Geometry: final body of the model. Coordinates: model frame, mm. Round coordinates to 2 decimals unless told otherwise and drop trailing zeros. Loops run counter-clockwise (first coordinate to the right, second up) from the corner with the lowest first, then second, coordinate; pieces in that order, holes last. Notation, with made-up numbers: (59.5, 2) - (75.5, 2) arc R25 cw to (75.5, 31) - close; hole circle Ø7 at (26.5, 39.25). An arc over 180 degrees is marked (long way). Use CSV: the item, a comma, the result in double quotes.
from build123d import *

# Parameters (mm, degrees)
SKETCH1_R           = 2.25
BOSS_EXTRUDE1_DEPTH = 2.15
SKETCH2_W           = 1.55
SKETCH2_H           = 4.8
CUT_EXTRUDE1_DEPTH  = 53


with BuildPart() as part:
    # Sketch1 → Boss-Extrude1 (new body)
    with BuildSketch(Plane.XY):
        with BuildLine():
            Line((2.398752887, -11.327345722), (26.384379929, -11.327345722))
            Line((26.384379929, -11.327345722), (26.384379929, 8.672654278))
            Line((26.384379929, 8.672654278), (26.024379959, 8.672654278))
            Line((26.024379959, 8.672654278), (24.744379959, 8.672654278))
            Line((24.744379959, 8.672654278), (24.744379959, 6.172654278))
            ThreePointArc((24.744379959, 6.172654278), (24.384379958, 5.812654278), (24.024379958, 6.172654278))
            Line((24.024379958, 6.172654278), (24.024379958, 8.672654278))
            Line((24.024379958, 8.672654278), (22.744379958, 8.672654278))
            Line((22.744379958, 8.672654278), (22.744379958, 6.172654278))
            ThreePointArc((22.744379958, 6.172654278), (22.384379957, 5.812654278), (22.024379957, 6.172654278))
            Line((22.024379957, 6.172654278), (22.024379957, 8.672654278))
            Line((22.024379957, 8.672654278), (20.744379957, 8.672654278))
            Line((20.744379957, 8.672654278), (20.744379957, 6.172654278))
            ThreePointArc((20.744379957, 6.172654278), (20.384379956, 5.812654278), (20.024379956, 6.172654278))
            Line((20.024379956, 6.172654278), (20.024379956, 8.672654278))
            Line((20.024379956, 8.672654278), (18.744379956, 8.672654278))
            Line((18.744379956, 8.672654278), (18.744379956, 6.172654278))
            ThreePointArc((18.744379956, 6.172654278), (18.384379955, 5.812654278), (18.024379955, 6.172654278))
            Line((18.024379955, 6.172654278), (18.024379955, 8.672654278))
            Line((18.024379955, 8.672654278), (16.744379955, 8.672654278))
            Line((16.744379955, 8.672654278), (16.744379955, 6.172654278))
            ThreePointArc((16.744379955, 6.172654278), (16.384379953, 5.812654278), (16.024379953, 6.172654278))
            Line((16.024379953, 6.172654278), (16.024379953, 8.672654278))
            Line((16.024379953, 8.672654278), (14.744379953, 8.672654278))
            Line((14.744379953, 8.672654278), (14.744379953, 6.172654278))
            ThreePointArc((14.744379953, 6.172654278), (14.384379952, 5.812654278), (14.024379952, 6.172654278))
            Line((14.024379952, 6.172654278), (14.024379952, 8.672654278))
            Line((14.024379952, 8.672654278), (12.744379952, 8.672654278))
            Line((12.744379952, 8.672654278), (12.744379952, 6.172654278))
            ThreePointArc((12.744379952, 6.172654278), (12.384379951, 5.812654278), (12.024379951, 6.172654278))
            Line((12.024379951, 6.172654278), (12.024379951, 8.672654278))
            Line((12.024379951, 8.672654278), (10.744379951, 8.672654278))
            Line((10.744379951, 8.672654278), (10.744379951, 6.172654278))
            ThreePointArc((10.744379951, 6.172654278), (10.38437995, 5.812654278), (10.02437995, 6.172654278))
            Line((10.02437995, 6.172654278), (10.02437995, 8.672654278))
            Line((10.02437995, 8.672654278), (8.74437995, 8.672654278))
            Line((8.74437995, 8.672654278), (8.74437995, 6.172654278))
            ThreePointArc((8.74437995, 6.172654278), (8.384379949, 5.812654278), (8.024379949, 6.172654278))
            Line((8.024379949, 6.172654278), (8.024379949, 8.672654278))
            Line((8.024379949, 8.672654278), (6.744379949, 8.672654278))
            Line((6.744379949, 8.672654278), (6.744379949, 6.172654278))
            ThreePointArc((6.744379949, 6.172654278), (6.384379947, 5.812654278), (6.024379947, 6.172654278))
            Line((6.024379947, 6.172654278), (6.024379947, 8.672654278))
            Line((6.024379947, 8.672654278), (4.744379947, 8.672654278))
            Line((4.744379947, 8.672654278), (4.744379947, 6.172654278))
            ThreePointArc((4.744379947, 6.172654278), (4.384379946, 5.812654278), (4.024379946, 6.172654278))
            Line((4.024379946, 6.172654278), (4.024379946, 8.672654278))
            Line((4.024379946, 8.672654278), (2.744379946, 8.672654278))
            Line((2.744379946, 8.672654278), (2.744379946, 6.172654278))
            ThreePointArc((2.744379946, 6.172654278), (2.384379945, 5.812654278), (2.024379945, 6.172654278))
            Line((2.024379945, 6.172654278), (2.024379945, 8.672654278))
            Line((2.024379945, 8.672654278), (0.744379945, 8.672654278))
            Line((0.744379945, 8.672654278), (0.744379945, 6.172654278))
            ThreePointArc((0.744379945, 6.172654278), (0.384379944, 5.812654278), (0.024379944, 6.172654278))
            Line((0.024379944, 6.172654278), (0.024379944, 8.672654278))
            Line((0.024379944, 8.672654278), (-1.255620056, 8.672654278))
            Line((-1.255620056, 8.672654278), (-1.255620056, 6.172654278))
            ThreePointArc((-1.255620056, 6.172654278), (-1.615620057, 5.812654278), (-1.975620057, 6.172654278))
            Line((-1.975620057, 6.172654278), (-1.975620057, 8.672654278))
            Line((-1.975620057, 8.672654278), (-3.255620057, 8.672654278))
            Line((-3.255620057, 8.672654278), (-3.255620057, 6.172654278))
            ThreePointArc((-3.255620057, 6.172654278), (-3.615620059, 5.812654278), (-3.975620059, 6.172654278))
            Line((-3.975620059, 6.172654278), (-3.975620059, 8.672654278))
            Line((-3.975620059, 8.672654278), (-5.255620059, 8.672654278))
            Line((-5.255620059, 8.672654278), (-5.255620059, 6.172654278))
            ThreePointArc((-5.255620059, 6.172654278), (-5.61562006, 5.812654278), (-5.97562006, 6.172654278))
            Line((-5.97562006, 6.172654278), (-5.97562006, 8.672654278))
            Line((-5.97562006, 8.672654278), (-7.25562006, 8.672654278))
            Line((-7.25562006, 8.672654278), (-7.25562006, 6.172654278))
            ThreePointArc((-7.25562006, 6.172654278), (-7.615620061, 5.812654278), (-7.975620061, 6.172654278))
            Line((-7.975620061, 6.172654278), (-7.975620061, 8.672654278))
            Line((-7.975620061, 8.672654278), (-9.255620061, 8.672654278))
            Line((-9.255620061, 8.672654278), (-9.255620061, 6.172654278))
            ThreePointArc((-9.255620061, 6.172654278), (-9.615620062, 5.812654278), (-9.975620062, 6.172654278))
            Line((-9.975620062, 6.172654278), (-9.975620062, 8.672654278))
            Line((-9.975620062, 8.672654278), (-11.255620062, 8.672654278))
            Line((-11.255620062, 8.672654278), (-11.255620062, 6.172654278))
            ThreePointArc((-11.255620062, 6.172654278), (-11.615620063, 5.812654278), (-11.975620063, 6.172654278))
            Line((-11.975620063, 6.172654278), (-11.975620063, 8.672654278))
            Line((-11.975620063, 8.672654278), (-13.255620063, 8.672654278))
            Line((-13.255620063, 8.672654278), (-13.255620063, 6.172654278))
            ThreePointArc((-13.255620063, 6.172654278), (-13.615620065, 5.812654278), (-13.975620065, 6.172654278))
            Line((-13.975620065, 6.172654278), (-13.975620065, 8.672654278))
            Line((-13.975620065, 8.672654278), (-15.255620065, 8.672654278))
            Line((-15.255620065, 8.672654278), (-15.255620065, 6.172654278))
            ThreePointArc((-15.255620065, 6.172654278), (-15.615620066, 5.812654278), (-15.975620066, 6.172654278))
            Line((-15.975620066, 6.172654278), (-15.975620066, 8.672654278))
            Line((-15.975620066, 8.672654278), (-17.255620066, 8.672654278))
            Line((-17.255620066, 8.672654278), (-17.255620066, 6.172654278))
            ThreePointArc((-17.255620066, 6.172654278), (-17.615620067, 5.812654278), (-17.975620067, 6.172654278))
            Line((-17.975620067, 6.172654278), (-17.975620067, 8.672654278))
            Line((-17.975620067, 8.672654278), (-19.255620067, 8.672654278))
            Line((-19.255620067, 8.672654278), (-19.255620067, 6.172654278))
            ThreePointArc((-19.255620067, 6.172654278), (-19.615620068, 5.812654278), (-19.975620068, 6.172654278))
            Line((-19.975620068, 6.172654278), (-19.975620068, 8.672654278))
            Line((-19.975620068, 8.672654278), (-21.255620068, 8.672654278))
            Line((-21.255620068, 8.672654278), (-21.255620068, 6.172654278))
            ThreePointArc((-21.255620068, 6.172654278), (-21.615620069, 5.812654278), (-21.975620069, 6.172654278))
            Line((-21.975620069, 6.172654278), (-21.975620069, 8.672654278))
            Line((-21.975620069, 8.672654278), (-23.255620069, 8.672654278))
            Line((-23.255620069, 8.672654278), (-23.255620069, 6.172654278))
            ThreePointArc((-23.255620069, 6.172654278), (-23.615620071, 5.812654278), (-23.975620071, 6.172654278))
            Line((-23.975620071, 6.172654278), (-23.975620071, 8.672654278))
            Line((-23.975620071, 8.672654278), (-25.615620071, 8.672654278))
            Line((-25.615620071, 8.672654278), (-25.615620071, -11.327345722))
            Line((-25.615620071, -11.327345722), (-1.621247113, -11.327345722))
            Line((-1.621247113, -11.327345722), (-1.621247113, -7.327345722))
            ThreePointArc((-1.621247113, -7.327345722), (0.373417474, -5.293808364), (2.398752887, -7.296800492))
            Line((2.398752887, -7.296800492), (2.398752887, -11.327345722))
        make_face()
        with Locations((-19.615620071, -5.327345722)):
            Circle(SKETCH1_R, mode=Mode.SUBTRACT)
        with Locations((-9.615620071, -5.327345722)):
            Circle(SKETCH1_R, mode=Mode.SUBTRACT)
        with Locations((10.384379929, -5.327345722)):
            Circle(SKETCH1_R, mode=Mode.SUBTRACT)
        with Locations((20.384379929, -5.327345722)):
            Circle(SKETCH1_R, mode=Mode.SUBTRACT)
    extrude(amount=BOSS_EXTRUDE1_DEPTH)

    # Sketch2 → Cut-Extrude1 (cut, through all)
    with BuildSketch(Plane.ZY.offset(25.615620071)):
        with Locations((1.375, 6.272654278)):
            Rectangle(SKETCH2_W, SKETCH2_H)
    extrude(amount=-CUT_EXTRUDE1_DEPTH, mode=Mode.SUBTRACT)


solid = part.part
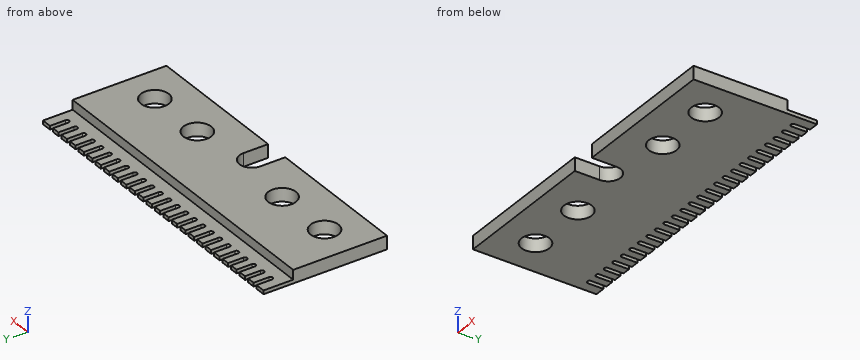
Item 1: Material intervals for line 1 (X direction, y = -6.25, z = 0.95); line 2 (X direction, y = -5.75, z = 0.25); line 3 (X direction, y = -5, z = 1.05), sorted ascending.
Final values:
line 1,"x = -25.62 to -21.67, -17.56 to -11.67, -7.56 to -1.32, 2.1 to 8.33, 12.44 to 18.33, 22.44 to 26.38"
line 2,"x = -25.62 to -21.83, -17.41 to -11.83, -7.41 to -0.89, 1.66 to 8.17, 12.59 to 18.17, 22.59 to 26.38"
line 3,"x = -25.62 to -21.84, -17.39 to -11.84, -7.39 to 8.16, 12.61 to 18.16, 22.61 to 26.38"
Item 2: Pin query (flat end, axial travel): P1, Ø2.5, axis at x = 10.38, y = -5.33, coming from the +Z side; P2, Ø1.4, axis at x = 3, y = 5, coming from the +Z side. Return the tip coordinate at first contact, or that it passes through.
Final values:
P1,"passes through"
P2,"stops at z = 0.6"
Item 3: Section B-B on z = 1.3. Return the cut outline in (x, y), plus the area to 3 significant figures.
Final values:
outline,"(-25.62, -11.33) - (-1.62, -11.33) - (-1.62, -7.33) arc R2.01 cw (long way) to (2.4, -7.3) - (2.4, -11.33) - (26.38, -11.33) - (26.38, 3.87) - (-25.62, 3.87) - close; hole circle Ø4.5 at (-19.62, -5.33); hole circle Ø4.5 at (-9.62, -5.33); hole circle Ø4.5 at (10.38, -5.33); hole circle Ø4.5 at (20.38, -5.33)"
area,"704 mm²"
Item 4: Section A-A on y = -9. Return the cut outline in (x, z), plus the area to 3 significant figures.
Final values:
outline,"(-25.62, 0) - (-1.62, 0) - (-1.62, 2.15) - (-25.62, 2.15) - close; (2.4, 0) - (26.38, 0) - (26.38, 2.15) - (2.4, 2.15) - close"
area,"103 mm²"
